Work out the finished part from the listing and answer in its coordinate system (mm). Give positions to 0.01 mm unless a question says otherwise; leave off trailing zeros. Write each loop counter-clockwise with the first axis right and the second up, starting at its lowest first coordinate (ties: lowest second). Pieces come first, ordered by that corner, then holes.
1) Find section B-B (z = 26). Determine the outline of the cut face in (x, y).
2) Straight lines are drawn through the part: probe 1 along Z at (x, y) = (-3, -3.75); probe 2 along Y at (x, z) = (0.25, 79); probe 3 along Z at (x, y) = (-1, -0.25). For each, find the intervals that lie inside material, in ascending order.
3) Given pin 1 Ø4 at (x, z) = (-3.5, 79) entering from +Y; pin 2 Ø3 at (y, z) = (4, 20) entering from -X; pin 3 Ø4 at (y, z) = (-2, 64.5) entering from -X, each flat-ended and moving along its own axis, determine where each tip first touches the part or whether it passes through.
4) Find section A-A (y = 0). Determine the outline of the cut face in (x, z).
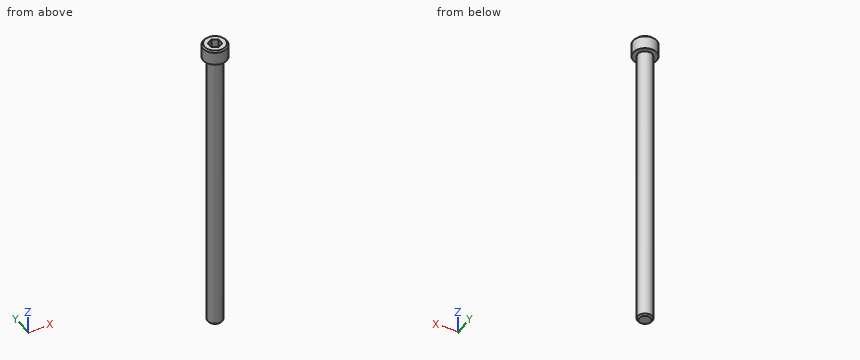
Autodesk Inventor part; units mm, degrees
ref_plane "YZ Plane" through (0, 0, 0) normal (1, 0, 0) x (0, 1, 0)
ref_plane "XZ Plane" through (0, 0, 0) normal (0, 1, 0) x (-1, 0, 0)
ref_plane "XY Plane" through (0, 0, 0) normal (0, 0, 1) x (1, 0, 0)
sketch "Sketch1" plane through (0, 0, 0) normal (0, 0, 1) x (1, 0, 0)
  circle A0 centre (0, 0) radius 4
  dimension "Diameter" = 8
extrude "Extrusion1" add sketch "Sketch1" along normal blind 160
sketch "Sketch2" plane through (0, 0, 160) normal (0, 0, 1) x (1, 0, 0)
  circle A0 centre (0, 0) radius 4
  circle A1 centre (0, 0) radius 6.5
  dimension "Head_Diameter" = 13
extrude "Extrusion2" add sketch "Sketch2" along normal blind 8 contours A0 | A1
sketch "Sketch3" plane through (0, 0, 168) normal (0, 0, 1) x (1, 0, 0)
  circle A0 centre (0, 0) radius 6.5
  circle A1 centre (0, 0) radius 3.4641 construction
  line L0 (0, 3.4641) -> (3, 1.7321)
  line L1 (3, -1.7321) -> (3, 1.7321)
  line L2 (0, 3.4641) -> (-3, 1.7321)
  line L3 (-3, -1.7321) -> (-3, 1.7321)
  line L4 (-3, -1.7321) -> (0, -3.4641)
  line L5 (3, -1.7321) -> (0, -3.4641)
  dimension "Hex_Width" = 6
extrude "Extrusion3" cut sketch "Sketch3" against normal blind 5 contours L0 L1 L5 L4 L3 L2
thread "Thread1"
chamfer "Chamfer1" distance 0.8 angle 45 2 edges at (-6.5, 0, 168) (-4, 0, 0)
equation "\"d9\" = ThreadLength"
equation "\"ThreadLength\" = 32"
properties part number "SCREW, SOCKET HD, P, 12.9, M8X1.25X160MM"
Results:
1. outline: circle Ø8 at (0, 0)
2. probe 1: z = 160 to 168
2. probe 2: y = -3.99 to 3.99
2. probe 3: z = 0 to 163
3. pin 1: stops at y = 3.71
3. pin 2: stops at x = -3.12
3. pin 3: stops at x = -4
4. outline: (-6.5, 160) - (-4, 160) - (-4, 0.8) - (-3.2, 0) - (3.2, 0) - (4, 0.8) - (4, 160) - (6.5, 160) - (6.5, 167.2) - (5.7, 168) - (3, 168) - (3, 163) - (-3, 163) - (-3, 168) - (-5.7, 168) - (-6.5, 167.2) - close
